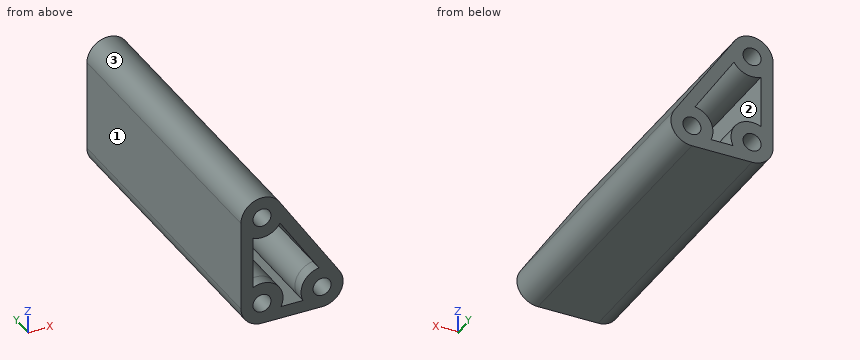
```python
from build123d import *
from build123d.topology import SkipClean

# Parameters (mm, degrees)
SKETCH1_R           = 1.5
BOSS_EXTRUDE1_DEPTH = 50
SHELL2_T            = -2
CUT_EXTRUDE1_DEPTH  = 54.219702176


with BuildPart() as part:
    # Sketch1 → Boss-Extrude1 (new body)
    with BuildSketch(Plane(origin=(0, 0, 0), x_dir=(1, 0, 0), z_dir=(0, 1, 0))):
        with BuildLine():
            Line((-11.236028054, 16.552141364), (-11.236028054, 1.552141364))
            ThreePointArc((-11.236028054, 1.552141364), (-8.641894712, -1.828599028), (-4.704939141, -0.197858636))
            Line((-4.704939141, -0.197858636), (5.169075286, 14.600123285))
            ThreePointArc((5.169075286, 14.600123285), (5.352827986, 18.19803576), (2.263971946, 20.052141364))
            Line((2.263971946, 20.052141364), (-7.736028054, 20.052141364))
            ThreePointArc((-7.736028054, 20.052141364), (-10.210901788, 19.027015098), (-11.236028054, 16.552141364))
        make_face()
        with Locations(Location((-7.736028054, 16.552141364, 0), (0, 0, 270))):
            Circle(SKETCH1_R, mode=Mode.SUBTRACT)
        with Locations(Location((2.263971946, 16.552141364, 0), (0, 0, 270))):
            Circle(SKETCH1_R, mode=Mode.SUBTRACT)
        with Locations(Location((-7.736028054, 1.552141364, 0), (0, 0, 270))):
            Circle(SKETCH1_R, mode=Mode.SUBTRACT)
    extrude(amount=BOSS_EXTRUDE1_DEPTH)

    # Shell2
    shell2_openings = [part.faces().sort_by_distance(p)[0] for p in [
        (-4.434629852, 50, -10.910758817),
    ]]
    offset(amount=SHELL2_T, openings=shell2_openings)

    # Sketch2 → Cut-Extrude1 (cut, through all)
    with SkipClean():  # the faces are left unmerged after this step: merging them gives an invalid solid
        with BuildSketch(Plane(origin=(0, 2, 0), x_dir=(1, 0, 0), z_dir=(0, 1, 0))):
            with BuildLine():
                Line((-9.236028054, 13.389863704), (-9.236028054, 4.714419024))
                ThreePointArc((-9.236028054, 4.714419024), (-6.72499281, 4.90293347), (-4.737288861, 3.357013451))
                Line((-4.737288861, 3.357013451), (1.75650333, 13.089125972))
                ThreePointArc((1.75650333, 13.089125972), (-0.822229583, 14.901274888), (-0.898305714, 18.052141364))
                Line((-0.898305714, 18.052141364), (-4.573750394, 18.052141364))
                ThreePointArc((-4.573750394, 18.052141364), (-5.26115432, 14.07726763), (-9.236028054, 13.389863704))
            make_face()
        extrude(amount=-CUT_EXTRUDE1_DEPTH, mode=Mode.SUBTRACT)


solid = part.part
```
Could you check a few things on this model? Use its own coordinates, in mm. Face numbers are marked on the shaded views. Give positions to 0.01 mm unless a question says otherwise; leave off trailing zeros. Write each loop counter-clockwise with the first axis right and the second up, starting at its lowest first coordinate (ties: lowest second). Pieces come first, ordered by that corner, then holes. Notation, with made-up numbers: (-28.5, 49.5) -> (5.5, 49.5) arc R24 ccw to (5.5, 76.5) -> close; hole circle Ø1 at (55, 38). An arc over 180 degrees is marked (long way). Write each question's results on one line, items separated by ' | '.
1. I want a section at D-D, the plane z = -17.25. Write out the boundary of the cut face in (x, y).
Check sheet entries:
outline: (-11.17, 0) -> (-9.06, 0) -> (-9.06, 50) -> (-11.17, 50) -> close; (-6.41, 0) -> (-4.31, 0) -> (-4.31, 50) -> (-6.41, 50) -> close; (-1.17, 0) -> (0.94, 0) -> (0.94, 50) -> (-1.17, 50) -> close; (3.59, 0) -> (5.69, 0) -> (5.69, 50) -> (3.59, 50) -> close
2. I want a section at C-C, the plane y = 9. Write out the boundary of the cut face in (x, z), then the cut area to 3 significant figures.
Check sheet entries:
outline: (-11.24, -16.55) arc R3.5 ccw to (-7.74, -20.05) -> (2.26, -20.05) arc R3.5 ccw to (5.17, -14.6) -> (-4.7, 0.2) arc R3.5 ccw to (-11.24, -1.55) -> close; hole circle Ø3 at (-7.74, -16.55); hole (-9.24, -13.39) arc R3.5 cw to (-4.57, -18.05) -> (-0.9, -18.05) arc R3.5 cw to (1.76, -13.09) -> (-4.74, -3.36) arc R3.5 cw to (-9.24, -4.71) -> close; hole circle Ø3 at (-7.74, -1.55); hole circle Ø3 at (2.26, -16.55) | area: 153 mm²
3. I need wall thicknesses on L1, parallel to Z at x = -7.75, y = 16; L2, parallel to Z at x = -7.25, y = 9; L3, parallel to X at y = 23.5, z = -17.5. Which ranges of each line are inside material? Lowest first, please.
Check sheet entries:
L1: z = -20.05 to -18.05, -15.05 to -13.05, -5.05 to -3.05, -0.05 to 1.95 | L2: z = -20.05 to -17.97, -15.13 to -13.09, -5.02 to -2.97, -0.13 to 1.91 | L3: x = -11.11 to -8.9, -6.57 to -4.37, -1.11 to 1.1, 3.43 to 5.63
4. If we mould it in two halves opening along X, with no side actions, what happens to the marked faces 1, 2 and 3? For each: released by +X, released by -X, zero draft, split by the parting line, or undercut.
Check sheet entries:
face 1: released by -X | face 2: undercut | face 3: split by the parting line
5. I want a section at A-A, the plane x = -3. Write out the boundary of the cut face in (y, z), then the cut area to 3 significant figures.
Check sheet entries:
outline: (0, -20.05) -> (50, -20.05) -> (50, -18.05) -> (0, -18.05) -> close; (0, -5.96) -> (50, -5.96) -> (50, -2.36) -> (0, -2.36) -> close | area: 280 mm²
6. Will these pins go through, and if not, where does the flat tip stop? pin 1 Ø4 at (x, z) = (2.26, -16.55) entering from -Y; pin 2 Ø4 at (x, y) = (-2.5, 35.5) entering from +Z; pin 3 Ø3 at (x, y) = (-9.5, 29) entering from +Z; pin 4 Ø9.5 at (y, z) = (29.5, -7) entering from +X.
Check sheet entries:
pin 1: stops at y = 0 | pin 2: stops at z = -0.11 | pin 3: stops at z = 1.94 | pin 4: stops at x = 3.27
7. I want a section at B-B, the plane z = -2.5. Write out the boundary of the cut face in (x, y).
Check sheet entries:
outline: (-11.24, 0) -> (-8.9, 0) -> (-8.9, 50) -> (-11.24, 50) -> close; (-6.57, 0) -> (-2.9, 0) -> (-2.9, 50) -> (-6.57, 50) -> close
